Work out the finished part from the listing and answer in its coordinate system (mm). Face numbers are marked on the shaded views. A direction names the side the tool comes from. Give positions to 0.01 mm unless a question says otherwise; leave off trailing zeros. Loops run counter-clockwise (first coordinate to the right, second up) from the corner with the lowest first, then second, coordinate; pieces in that order, holes last.
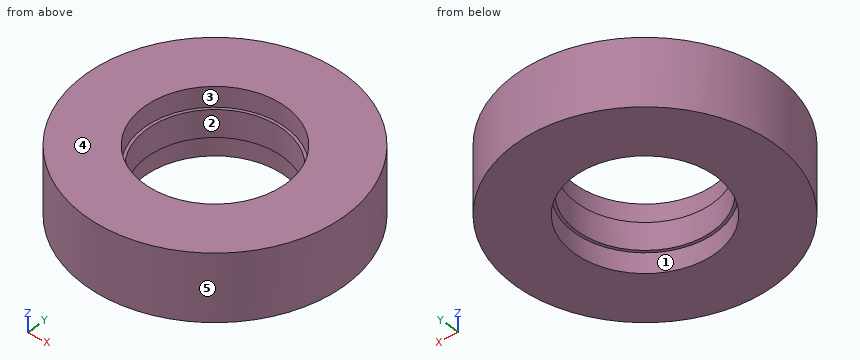
Autodesk Inventor part; units mm, degrees
ref_plane "YZ Plane" through (0, 0, 0) normal (1, 0, 0) x (0, 1, 0)
ref_plane "XZ Plane" through (0, 0, 0) normal (0, 1, 0) x (-1, 0, 0)
ref_plane "XY Plane" through (0, 0, 0) normal (0, 0, 1) x (1, 0, 0)
sketch "Sketch1" plane through (0, 0, 0) normal (0, 0, 1) x (1, 0, 0)
  circle A0 centre (0, 0) radius 19.05
  circle A1 centre (0, 0) radius 18.288
  dimension "d6" = 38.1
  dimension "d14" = 36.576
extrude "Extrusion1" add sketch "Sketch1" along normal mid plane 7.28
sketch "Sketch2" plane through (0, 0, 3.64) normal (0, 0, 1) x (1, 0, 0)
  circle A0 centre (0, 0) radius 34.925
  circle A1 centre (0, 0) radius 19.05
  dimension "d10" = 69.85
extrude "Extrusion2" add sketch "Sketch2" against normal blind 12.7
mirror "Mirror1" about plane through (0, 0, 0) normal (0, 0, 1) of "Extrusion2"
equation "\"d7\" = Length"
equation "\"Length\" = 7.28"
properties part number "Drift1615"
Q1. Section C-C on z = -7.25 is taken. Give the vertices of the cut face in (x, y) (3 decimals), plus the area to 3 significant figures.
Q2. Determine the mould class of the marked faces 3, 4 and 5 for opening direction X: +X half, -X half, draft (parallel to the pull), parting line (faces both ways), or undercut.
Q3. Section D-D on y = -26 is taken. Give the vertices of the cut face in (x, z).
Q4. Which of the six approach directions +Z, -Z, +X, -X, +Y, -Y give full straight-line access (tool end or side, diameter ignored) to the marked faces 1 and 2?
Q5. Given pin 1 (1 mm diameter, centred on y = 10.5, z = -1, fed in from -X); pin 2 (1.5 mm diameter, centred on y = 9.5, z = -5, fed in from -X); pin 3 (10 mm diameter, centred on x = 21, z = 6, fed in from -Y); pin 4 (23 mm diameter, centred on x = 0, y = 0, fed in from +Z), each flat-ended and moving along its own axis, determine where each tip first touches the part or whether it passes through.
Q6. Section A-A on x = 0 is taken. Give the vertices of the cut face in (y, z) (3 decimals), plus the area to 3 significant figures.
Q7. Consider line 1 along Y through (x, z) = (0, 7.55) (3 decimals); line 2 along Y through (x, z) = (-2, 7.25); line 3 along X through (y, z) = (-4.5, 0). Determine where each line is inside the solid, lowest interval first.
Check result:
1. outline: circle Ø69.85 at (0, 0); hole circle Ø38.1 at (0, 0)
1. area: 2,690 mm2
2. face 3: undercut
2. face 4: draft
2. face 5: parting line
3. outline: (-23.32, -9.06) - (23.32, -9.06) - (23.32, 9.06) - (-23.32, 9.06) - close
4. face 1: -Z
4. face 2: +Z, -Z
5. pin 1: stops at x = -33.46
5. pin 2: stops at x = -33.81
5. pin 3: stops at y = -31.04
5. pin 4: passes through
6. outline: (-34.925, -9.06) - (-19.05, -9.06) - (-19.05, -3.64) - (-18.288, -3.64) - (-18.288, 3.64) - (-19.05, 3.64) - (-19.05, 9.06) - (-34.925, 9.06) - close; (18.288, -3.64) - (19.05, -3.64) - (19.05, -9.06) - (34.925, -9.06) - (34.925, 9.06) - (19.05, 9.06) - (19.05, 3.64) - (18.288, 3.64) - close
6. area: 586 mm2
7. line 1: y = -34.925 to -19.05, 19.05 to 34.925
7. line 2: y = -34.87 to -18.94, 18.94 to 34.87
7. line 3: x = -34.63 to -17.73, 17.73 to 34.63
